Solid Edge part; units mm, degrees
sketch "Sketch1" plane through (0, 0, 0) normal (1, 0, 0) x (0, 1, 0)
  line L0 (-16.4084, 0) -> (-16.4084, 11.176)
  arc A0 (-12.0904, 15.494) -> (-16.4084, 11.176) centre (-12.0904, 11.176) ccw
  line L1 (-12.0904, 15.494) -> (12.0904, 15.494)
  arc A1 (12.0904, 15.494) -> (16.4084, 11.176) centre (12.0904, 11.176) cw
  line L2 (16.4084, 11.176) -> (16.4084, 0)
  line L3 (16.4084, 0) -> (-16.4084, 0)
extrude "Protrusion1" add sketch "Sketch1" along normal blind 58.801
sketch "Sketch2" plane through (29.4005, 0, 0) normal (0, 0, -1) x (1, 0, 0)
  circle A0 centre (-27.0891, -7.239) radius 0.254
  circle A1 centre (-27.0891, 7.239) radius 0.254
extrude "ExtrudedProtrusion_2" add sketch "Sketch2" along normal blind 13.4112
sketch "Sketch3" plane through (29.4005, 0, 0) normal (0, 0, -1) x (0, -1, 0)
  circle A0 centre (-7.5057, 0) radius 1.6002
  circle A1 centre (7.5057, 0) radius 1.6002
extrude "Cutout1" cut sketch "Sketch3" against normal through all
Geometry: final body of the model. Coordinates: model frame, mm. Give positions to 0.01 mm unless a question says otherwise; leave off trailing zeros. Write each loop counter-clockwise with the first axis right and the second up, starting at its lowest first coordinate (ties: lowest second). Pieces come first, ordered by that corner, then holes. Notation, with made-up numbers: (-26, 30.5) -> (-20, 30.5) arc R28 cw to (-20, 64.5) -> close; hole circle Ø3 at (79, 8). An arc over 180 degrees is marked (long way). Answer as a JSON object with one key per item and string values.
1. Cut plane C-C on x = 48. Output: boundary loops of the cut face in (y, z), and give its area (3 significant figures).
Ans:
{"outline": "(-16.41, 0) -> (16.41, 0) -> (16.41, 11.18) arc R4.32 ccw to (12.09, 15.49) -> (-12.09, 15.49) arc R4.32 ccw to (-16.41, 11.18) -> close", "area": "500 mm^2"}
2. Mould query, pull axis X, two halves, no side actions, for faces 1 (the cylindrical face through (30.963, 7.853, 7.639)), 2 (the cylindrical face through (30.963, -7.159, 7.639)), 3 (the flat face through (0, 0, 8)), 4 (the flat face through (29, -16.408, 6)). Classes: pulls with the +X half, pulls with the -X half, needs draft (parallel to the pull), parting line crosses it, or undercut.
Ans:
{"face 1": "undercut", "face 2": "undercut", "face 3": "pulls with the -X half", "face 4": "needs draft"}
3. Cut plane A-A on y = 8.5. Output: boundary loops of the cut face in (x, z), and give its area (3 significant figures).
Ans:
{"outline": "(0, 0) -> (28.15, 0) -> (28.15, 15.49) -> (0, 15.49) -> close; (30.65, 0) -> (58.8, 0) -> (58.8, 15.49) -> (30.65, 15.49) -> close", "area": "872 mm^2"}
4. Cut plane B-B on z = 13.75. Output: boundary loops of the cut face in (x, y).
Ans:
{"outline": "(0, -15.56) -> (58.8, -15.56) -> (58.8, 15.56) -> (0, 15.56) -> close; hole circle Ø3.2 at (29.4, -7.51); hole circle Ø3.2 at (29.4, 7.51)"}
5. Ray query, probe 1 along Y at (x, z) = (30, 11); probe 2 along Z at (x, y) = (26, -11); probe 3 along Y at (x, z) = (30.5, 5). Return the intervals inside material, ascending. Write a range as from..to.
Ans:
{"probe 1": "y = -16.41..-8.99, -6.02..6.02, 8.99..16.41", "probe 2": "z = 0..15.49", "probe 3": "y = -16.41..-8.67, -6.34..6.34, 8.67..16.41"}
6. Contact query for flat-ended pins moving along their axis: pin 1 (1 mm diameter, centred on x = 50.5, y = 11.5, fed in from -Z); pin 2 (1.9 mm diameter, centred on x = 29.4, y = 7.51, fed in from +Z). Output: stop coordinate, or through.
Ans:
{"pin 1": "stops at z = 0", "pin 2": "passes through"}
7. Cut plane D-D on y = -11. Output: boundary loops of the cut face in (x, z), and give its area (3 significant figures).
Ans:
{"outline": "(0, 0) -> (58.8, 0) -> (58.8, 15.49) -> (0, 15.49) -> close", "area": "911 mm^2"}
